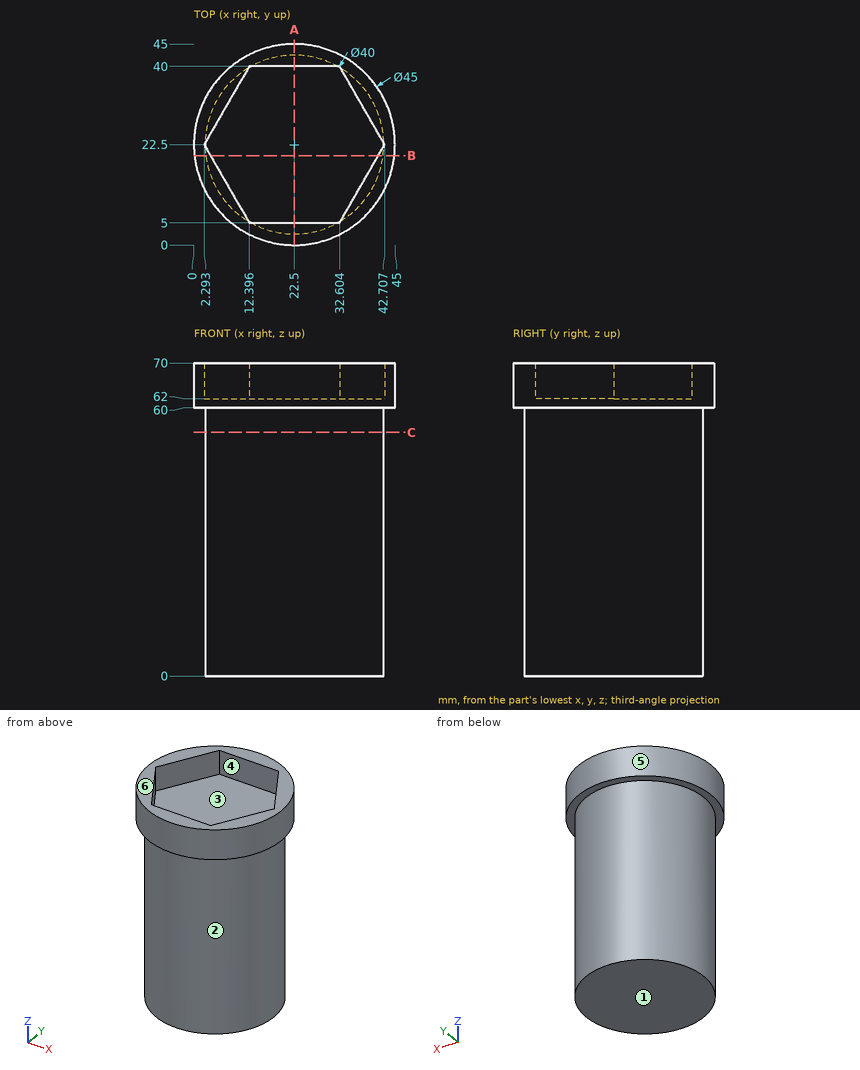
For this review, use the dimensioned drawing (mm, ordinates from the lowest corner) and the shaded views. A direction names the side the tool comes from. Round coordinates to 2 decimals unless told otherwise and drop trailing zeros. Order: outer loops, then holes, each group sorted by start corner. A loop starts at its lowest first (then second) coordinate and runs counter-clockwise, first axis right, second up. Notation, with made-up numbers: M -28,78 L 6,78 A19 cw 6,104 Z; hole C 26.25,-12.75 d9. An arc over 180 degrees is marked long. Write each question's results on one line, items separated by ' | '. Start each with the question number.
1. Draft analysis for pull direction Y (two halves, no side actions). For the marked faces 4, 5 and 6, state which applies: pulls with the +Y half, pulls with the -Y half, needs draft (parallel to the pull), parting line crosses it, or undercut.
2. Add section A-A (x = 22.5). State the section outline as (y, z) points, then the cut area to 3 significant figures.
3. Tool access review of the marked faces 1, 2 and 3: name each direction out of +Z, -Z, +X, -X, +Y, -Y from which nothing blocks a thin tool from reaching the whole face with its end or side.
4. Add section B-B (y = 20). State the section outline as (x, z) points.
5. Clearance check with flat-ended pins moving along their axes: pin 1 Ø8 at (y, z) = (8.5, 54) entering from +X; pin 2 Ø1.5 at (x, y) = (6, 9) entering from -Z; pin 3 Ø6 at (x, z) = (11, 39.5) entering from -Y. State where each tip first meets the part, or that it passes through.
6. Add section C-C (z = 54.5). State the section outline as (x, y) points, then the cut area to 3 significant figures.
7. To check wall thickness, follow L1, parallel to Z at x = 42, y = 21.5; L2, parallel to Y at x = 30, z = 64; L3, parallel to Z at x = 41.5, y = 12. State the ranges of each line that lie inside material, in increasing order. Write a range as [from, to].
Output values:
1) face 4: undercut | face 5: parting line crosses it | face 6: needs draft
2) outline: M 0,60 L 2.5,60 L 2.5,0 L 42.5,0 L 42.5,60 L 45,60 L 45,70 L 40,70 L 40,62 L 5,62 L 5,70 L 0,70 Z | area: 2,570 mm^2
3) face 1: -Z, +X, -X, +Y, -Y | face 2: -Z | face 3: +Z
4) outline: M 0.14,60 L 2.66,60 L 2.66,0 L 42.34,0 L 42.34,60 L 44.86,60 L 44.86,70 L 41.26,70 L 41.26,62 L 3.74,62 L 3.74,70 L 0.14,70 Z
5) pin 1: x = 39.82 | pin 2: z = 60 | pin 3: y = 4.4
6) outline: C 22.5,22.5 d40 | area: 1,260 mm^2
7) L1: [0, 62] | L2: [1.29, 5], [40, 43.71] | L3: [60, 70]
